from build123d import *

# Parameters (mm, degrees)
SKETCH_1_R          = 6.45
SKETCH_1_R_2        = 4.2
EXTRUDE_1_DEPTH     = 2
SKETCH_2_R          = 4.2
EXTRUDE_3_DEPTH     = 2.4
SKETCH_3_R          = 1.4
CUT_EXTRUDE_1_DEPTH = 10


with BuildPart() as part:
    # 스케치1 → 보스-돌출1 (new body)
    with BuildSketch(Plane(origin=(0, 0, 0), x_dir=(1, 0, 0), z_dir=(0, 1, 0))):
        Circle(SKETCH_1_R)
        Circle(SKETCH_1_R_2, mode=Mode.SUBTRACT)
    extrude(amount=EXTRUDE_1_DEPTH)

    # 스케치2 → 보스-돌출3 (add)
    with BuildSketch(Plane.XZ):
        with BuildLine():
            Line((-14, 8.6), (14, 8.6))
            ThreePointArc((14, 8.6), (22.6, 0), (14, -8.6))
            Line((14, -8.6), (-14, -8.6))
            ThreePointArc((-14, -8.6), (-22.6, 0), (-14, 8.6))
        make_face()
        Circle(SKETCH_2_R, mode=Mode.SUBTRACT)
    extrude(amount=EXTRUDE_3_DEPTH)

    # 스케치3 → 컷-돌출1 (cut)
    with BuildSketch(Plane.XZ.offset(2.4)):
        with Locations((-21, 0)):
            Circle(SKETCH_3_R)
    cut_extrude_1 = extrude(amount=-CUT_EXTRUDE_1_DEPTH, mode=Mode.SUBTRACT)

    # 대칭 복사1: 컷-돌출1 across plane
    add(cut_extrude_1.mirror(Plane(origin=(0, 0, 0), x_dir=(0, 0, 1), z_dir=(1, 0, 0))), mode=Mode.SUBTRACT)


solid = part.part
Geometry check sheet. Reference: the model listing, model coordinates, mm. Round coordinates to 2 decimals unless told otherwise and drop trailing zeros. Loops run counter-clockwise (first coordinate to the right, second up) from the corner with the lowest first, then second, coordinate; pieces in that order, holes last.
Item 1: Mould release check, pull along X, two halves, no side actions. Record for faces 1 (the cylindrical face through (19.71, -1.22, -0.54)), 2 (the cylindrical face through (-1.398, 0.986, 6.297)), 3 (the flat face through (0, -1, -8.6)): pulls with the +X half, pulls with the -X half, needs draft (parallel to the pull), parting line crosses it, or undercut.
Item 2: Cross-section at C-C on z = 3.5. Record the boundary of the cut face in (x, y), then the cut area to 3 significant figures.
Item 3: Gauge pin test, flat ends, axial feed: pin 1 (1 mm diameter, centred on y = 0, z = -3, fed in from +X); pin 2 (6 mm diameter, centred on x = 13.5, z = 7, fed in from +Y); pin 3 (1 mm diameter, centred on y = -0.5, z = -1.5, fed in from +X). Record the tip position at first contact, or that the pin passes through.
Item 4: Cross-section at B-B on y = -1.7. Record the boundary of the cut face in (x, z).
Item 5: Thickness scan on line 1 (Z direction, x = 0, y = -1.1); line 2 (Y direction, x = 9, z = -1.5); line 3 (Z direction, x = 0, y = 0.9). Record the ranges inside material, lowest first.
Item 6: Cross-section at D-D on z = -5.5. Record the boundary of the cut face in (x, y), then the cut area to 3 significant figures.
Item 7: Cross-section at A-A on x = 0. Record the boundary of the cut face in (y, z).
Answer sheet:
1. face 1: undercut
1. face 2: parting line crosses it
1. face 3: needs draft
2. outline: (-21.86, -2.4) - (-2.32, -2.4) - (-2.32, 2) - (-5.42, 2) - (-5.42, 0) - (-21.86, 0) - close; (2.32, -2.4) - (21.86, -2.4) - (21.86, 0) - (5.42, 0) - (5.42, 2) - (2.32, 2) - close
2. area: 106 mm2
3. pin 1: stops at x = 22.23
3. pin 2: stops at y = 0
3. pin 3: stops at x = 22.54
4. outline: (-14, -8.6) - (14, -8.6) arc R8.6 ccw to (14, 8.6) - (-14, 8.6) arc R8.6 ccw to start; hole circle Ø2.8 at (-21, 0); hole circle Ø8.4 at (0, 0); hole circle Ø2.8 at (21, 0)
5. line 1: z = -8.6 to -4.2, 4.2 to 8.6
5. line 2: y = -2.4 to 0
5. line 3: z = -6.45 to -4.2, 4.2 to 6.45
6. outline: (-20.61, -2.4) - (20.61, -2.4) - (20.61, 0) - (3.37, 0) - (3.37, 2) - (-3.37, 2) - (-3.37, 0) - (-20.61, 0) - close
6. area: 112 mm2
7. outline: (-2.4, -8.6) - (0, -8.6) - (0, -6.45) - (2, -6.45) - (2, -4.2) - (-2.4, -4.2) - close; (-2.4, 4.2) - (2, 4.2) - (2, 6.45) - (0, 6.45) - (0, 8.6) - (-2.4, 8.6) - close
